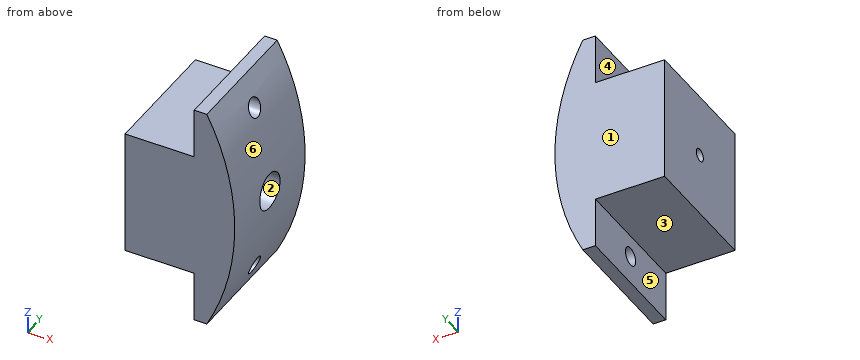
```python
from build123d import *

# Parameters (mm, degrees)
SKETCH2_W               = 13.97
SKETCH2_H               = 25.4
BOSS_EXTRUDE1_DEPTH     = 25.4
CUT_EXTRUDE2_REACH      = 42.718
CUT_EXTRUDE2_END_RADIUS = 49.2125
SKETCH4_R               = 1.27
CUT_EXTRUDE4_START      = -8.171649
SKETCH11_R              = 3.6576
CUT_EXTRUDE4_DEPTH      = 12.7
CUT_EXTRUDE5_REACH      = 61.913
CUT_EXTRUDE5_END_RADIUS = 49.2125
SKETCH15_R              = 1.8288


with BuildPart() as part:
    # Sketch2 → Boss-Extrude1 (new body)
    with BuildSketch(Plane(origin=(0, 0, 0), x_dir=(1, 0, 0), z_dir=(0, 1, 0))):
        with Locations((34.055850798, 0)):
            Rectangle(SKETCH2_W, SKETCH2_H)
        Polygon((43.580850798, -22.86), (43.580850798, 22.86), (41.040850798, 22.86), (41.040850798, 12.7), (41.040850798, -12.7), (41.040850798, -22.86), align=None)
        with BuildLine():
            Line((43.580850798, 22.86), (43.580850798, -22.86))
            ThreePointArc((43.580850798, -22.86), (49.2125, 0), (43.580850798, 22.86))
        make_face()
    extrude(amount=BOSS_EXTRUDE1_DEPTH)

    # Cut-Extrude2: up to this cylinder (the profile starts inside it)
    cut_extrude2_end = Plane(origin=(0, 12.7, 0), z_dir=(0, -1, 0)) * Cylinder(CUT_EXTRUDE2_END_RADIUS, 184.861, mode=Mode.PRIVATE)
    # Sketch4 → Cut-Extrude2 (cut, up to the surface)
    with BuildSketch(Plane.ZY.offset(-27.070850798), mode=Mode.PRIVATE) as cut_extrude2_sk1:
        with Locations((0, 12.7)):
            Circle(SKETCH4_R)
    cut_extrude2_tool1 = extrude(cut_extrude2_sk1.sketch, amount=-CUT_EXTRUDE2_REACH, mode=Mode.PRIVATE) & cut_extrude2_end
    add(cut_extrude2_tool1.solids().sort_by_distance((27.070851, 12.7, 0))[0], mode=Mode.SUBTRACT)

    # Sketch11 → Cut-Extrude4 (cut)
    with BuildSketch(Plane.ZY.offset(-41.040850798).offset(CUT_EXTRUDE4_START)):
        with Locations(Location((0, 12.7, 0), (0, 0, 180))):
            Circle(SKETCH11_R)
    extrude(amount=CUT_EXTRUDE4_DEPTH, mode=Mode.SUBTRACT)

    # Cut-Extrude5: up to this cylinder (the profile starts inside it)
    cut_extrude5_end = Plane(origin=(0, 12.7, 0), z_dir=(0, -1, 0)) * Cylinder(CUT_EXTRUDE5_END_RADIUS, 224.803334, mode=Mode.PRIVATE)
    # Sketch15 → Cut-Extrude5 (cut, up to the surface)
    with BuildSketch(Plane(origin=(0, 0, 0), x_dir=(0, 0, -1), z_dir=(1, 0, 0)), mode=Mode.PRIVATE) as cut_extrude5_sk1:
        with BuildLine():
            ThreePointArc((-18.9738, 12.7), (-17.145, 10.8712), (-15.3162, 12.7))
            Line((-15.3162, 12.7), (-18.9738, 12.7))
        make_face()
    cut_extrude5_tool1 = extrude(cut_extrude5_sk1.sketch, amount=CUT_EXTRUDE5_REACH, mode=Mode.PRIVATE) & cut_extrude5_end
    add(cut_extrude5_tool1.solids().sort_by_distance((0, 11.923833, 17.145))[0], mode=Mode.SUBTRACT)
    # Sketch15 → Cut-Extrude5 (cut, up to the surface)
    with BuildSketch(Plane(origin=(0, 0, 0), x_dir=(0, 0, -1), z_dir=(1, 0, 0)), mode=Mode.PRIVATE) as cut_extrude5_sk2:
        with BuildLine():
            Line((-18.9738, 12.7), (-15.3162, 12.7))
            ThreePointArc((-15.3162, 12.7), (-17.145, 14.5288), (-18.9738, 12.7))
        make_face()
    cut_extrude5_tool2 = extrude(cut_extrude5_sk2.sketch, amount=CUT_EXTRUDE5_REACH, mode=Mode.PRIVATE) & cut_extrude5_end
    add(cut_extrude5_tool2.solids().sort_by_distance((0, 13.476167, 17.145))[0], mode=Mode.SUBTRACT)
    # Sketch15 → Cut-Extrude5 (cut, up to the surface)
    with BuildSketch(Plane(origin=(0, 0, 0), x_dir=(0, 0, -1), z_dir=(1, 0, 0)), mode=Mode.PRIVATE) as cut_extrude5_sk3:
        with Locations(Location((17.145, 12.7, 0), (0, 0, 180))):
            Circle(SKETCH15_R)
    cut_extrude5_tool3 = extrude(cut_extrude5_sk3.sketch, amount=CUT_EXTRUDE5_REACH, mode=Mode.PRIVATE) & cut_extrude5_end
    add(cut_extrude5_tool3.solids().sort_by_distance((0, 12.7, -17.145))[0], mode=Mode.SUBTRACT)


solid = part.part
```
Check sheet for the modelled part. Datum: model origin and axes. Units: mm. Face numbers are marked on the shaded views. A direction names the side the tool comes from. Round coordinates to 2 decimals unless told otherwise and drop trailing zeros. Order: outer loops, then holes, each group sorted by start corner. A loop starts at its lowest first (then second) coordinate and runs counter-clockwise, first axis right, second up.
1) Scan lines: line 1 (Y direction, x = 45.25, z = 0); line 2 (Z direction, x = 37.75, y = 2.75); line 3 (Y direction, x = 42.75, z = -2). Record each from-to range of solid material in increasing order.
2) Section check A-A (x = 42.75). Record the boundary of the cut face in (y, z) (3 decimals), and give its area (3 significant figures).
3) Section check B-B (z = 0). Record the boundary of the cut face in (x, y), and give its area (3 significant figures).
4) Go/stop test with flat-tipped pins: pin 1 Ø3 at (y, z) = (18.5, -20) entering from -X; pin 2 Ø3.5 at (y, z) = (13.5, -1) entering from +X. Record where each tip stops, or that it passes through.
5) Mould release check, pull along Z, two halves, no side actions. Record for the marked faces 1, 2 and 3: +Z half, -Z half, draft (parallel to the pull), parting line (faces both ways), or undercut.
6) Section check C-C (y = 12.7). Record the boundary of the cut face in (x, z) (1 decimal).
7) Section check D-D (x = 33.5). Record the boundary of the cut face in (y, z), and give its area (3 significant figures).
8) Tool access check on the marked faces 4, 5 and 6. Record the directions out of +Z, -Z, +X, -X, +Y, -Y that give a thin tool (end or side, any length) a straight path to the whole face; none if there is none.
Result:
1. line 1: y = 0 to 9.04, 16.36 to 25.4
1. line 2: z = -12.7 to 12.7
1. line 3: y = 0 to 9.64, 15.76 to 25.4
2. outline: (0, -22.86) - (25.4, -22.86) - (25.4, 22.86) - (0, 22.86) - close; hole circle Ø7.315 at (12.7, 0); hole circle Ø3.658 at (12.7, -17.145); hole circle Ø3.658 at (12.7, 17.145)
2. area: 1,100 mm2
3. outline: (27.07, 0) - (49.21, 0) - (49.21, 9.04) - (36.51, 9.04) - (36.51, 11.43) - (27.07, 11.43) - close; (27.07, 13.97) - (36.51, 13.97) - (36.51, 16.36) - (49.21, 16.36) - (49.21, 25.4) - (27.07, 25.4) - close
3. area: 446 mm2
4. pin 1: stops at x = 41.04
4. pin 2: stops at x = 36.51
5. face 1: draft
5. face 2: undercut
5. face 3: -Z half
6. outline: (27.1, -12.7) - (41, -12.7) - (41, -15.3) - (46.8, -15.3) arc R49.2 ccw to (49.1, -3.7) - (36.5, -3.7) - (36.5, -1.3) - (27.1, -1.3) - close; (27.1, 1.3) - (36.5, 1.3) - (36.5, 3.7) - (49.1, 3.7) arc R49.2 ccw to (46.8, 15.3) - (41, 15.3) - (41, 12.7) - (27.1, 12.7) - close; (41, -22.9) - (43.6, -22.9) arc R49.2 ccw to (45.4, -19) - (41, -19) - close; (41, 19) - (45.4, 19) arc R49.2 ccw to (43.6, 22.9) - (41, 22.9) - close
7. outline: (0, -12.7) - (25.4, -12.7) - (25.4, 12.7) - (0, 12.7) - close; hole circle Ø2.54 at (12.7, 0)
7. area: 640 mm2
8. face 4: +Z, -X, +Y, -Y
8. face 5: -Z, -X, +Y, -Y
8. face 6: +X, +Y, -Y
